Read the model definition and answer for the solid it produces. Units are mm, in the model's axes. A direction names the side the tool comes from. Coordinates: 2 decimals unless noted, no trailing zeros. Order: outer loops, then holes, each group sorted by start corner. A loop starts at its lowest first (then second) coordinate and runs counter-clockwise, first axis right, second up.
```python
from build123d import *

# Parameters (mm, degrees)
BOSS_EXTRUDE1_DEPTH    = 2
FILLET1_R              = 1
SKETCH2_R              = 1.65
BOSS_EXTRUDE2_DEPTH    = 2
CONVERT_SOLID1_START   = -25
CONVERT_SOLID1_DEPTH   = 25
CONVERT_SOLID1_2_DEPTH = 25


# Read off the part's stored shape, not the designer's step: Convert-Solid1
with BuildPart() as part:
    # Sketch1 → Boss-Extrude1 (new body)
    with BuildSketch(Plane(origin=(0, 0, 0), x_dir=(1, 0, 0), z_dir=(0, 1, 0))):
        with BuildLine():
            Line((51, 12.5), (47.9, 12.5))
            ThreePointArc((47.9, 12.5), (46.4, 11), (44.9, 12.5))
            Line((44.9, 12.5), (41.7, 12.5))
            ThreePointArc((41.7, 12.5), (40.2, 11), (38.7, 12.5))
            Line((38.7, 12.5), (35.5, 12.5))
            ThreePointArc((35.5, 12.5), (34, 11), (32.5, 12.5))
            Line((32.5, 12.5), (29.3, 12.5))
            ThreePointArc((29.3, 12.5), (27.8, 11), (26.3, 12.5))
            Line((26.3, 12.5), (23.1, 12.5))
            ThreePointArc((23.1, 12.5), (21.6, 11), (20.1, 12.5))
            Line((20.1, 12.5), (16.9, 12.5))
            ThreePointArc((16.9, 12.5), (15.4, 11), (13.9, 12.5))
            Line((13.9, 12.5), (10.7, 12.5))
            ThreePointArc((10.7, 12.5), (9.2, 11), (7.7, 12.5))
            Line((7.7, 12.5), (0, 12.5))
            Line((0, 12.5), (0, 0))
            Line((0, 0), (4.7, 0))
            Line((4.7, 0), (4.7, 1.5))
            ThreePointArc((4.7, 1.5), (6.2, 3), (7.7, 1.5))
            Line((7.7, 1.5), (7.7, 0))
            Line((7.7, 0), (10.9, 0))
            Line((10.9, 0), (10.9, 1.5))
            ThreePointArc((10.9, 1.5), (12.4, 3), (13.9, 1.5))
            Line((13.9, 1.5), (13.9, 0))
            Line((13.9, 0), (17.1, 0))
            Line((17.1, 0), (17.1, 1.5))
            ThreePointArc((17.1, 1.5), (18.6, 3), (20.1, 1.5))
            Line((20.1, 1.5), (20.1, 0))
            Line((20.1, 0), (23.3, 0))
            Line((23.3, 0), (23.3, 1.5))
            ThreePointArc((23.3, 1.5), (24.8, 3), (26.3, 1.5))
            Line((26.3, 1.5), (26.3, 0))
            Line((26.3, 0), (29.5, 0))
            Line((29.5, 0), (29.5, 1.5))
            ThreePointArc((29.5, 1.5), (31, 3), (32.5, 1.5))
            Line((32.5, 1.5), (32.5, 0))
            Line((32.5, 0), (35.7, 0))
            Line((35.7, 0), (35.7, 1.5))
            ThreePointArc((35.7, 1.5), (37.2, 3), (38.7, 1.5))
            Line((38.7, 1.5), (38.7, 0))
            Line((38.7, 0), (41.9, 0))
            Line((41.9, 0), (41.9, 1.5))
            ThreePointArc((41.9, 1.5), (43.4, 3), (44.9, 1.5))
            Line((44.9, 1.5), (44.9, 0))
            Line((44.9, 0), (46.5, 0))
            ThreePointArc((46.5, 0), (49.681980515, 1.318019485), (51, 4.5))
            Line((51, 4.5), (51, 12.5))
        make_face()
        with BuildLine():
            ThreePointArc((44.9, 12.5), (46.4, 14), (47.9, 12.5))
            Line((47.9, 12.5), (51, 12.5))
            Line((51, 12.5), (51, 20.5))
            ThreePointArc((51, 20.5), (49.681980515, 23.681980515), (46.5, 25))
            Line((46.5, 25), (44.9, 25))
            Line((44.9, 25), (44.9, 23.5))
            ThreePointArc((44.9, 23.5), (43.4, 22), (41.9, 23.5))
            Line((41.9, 23.5), (41.9, 25))
            Line((41.9, 25), (38.7, 25))
            Line((38.7, 25), (38.7, 23.5))
            ThreePointArc((38.7, 23.5), (37.2, 22), (35.7, 23.5))
            Line((35.7, 23.5), (35.7, 25))
            Line((35.7, 25), (32.5, 25))
            Line((32.5, 25), (32.5, 23.5))
            ThreePointArc((32.5, 23.5), (31, 22), (29.5, 23.5))
            Line((29.5, 23.5), (29.5, 25))
            Line((29.5, 25), (26.3, 25))
            Line((26.3, 25), (26.3, 23.5))
            ThreePointArc((26.3, 23.5), (24.8, 22), (23.3, 23.5))
            Line((23.3, 23.5), (23.3, 25))
            Line((23.3, 25), (20.1, 25))
            Line((20.1, 25), (20.1, 23.5))
            ThreePointArc((20.1, 23.5), (18.6, 22), (17.1, 23.5))
            Line((17.1, 23.5), (17.1, 25))
            Line((17.1, 25), (13.9, 25))
            Line((13.9, 25), (13.9, 23.5))
            ThreePointArc((13.9, 23.5), (12.4, 22), (10.9, 23.5))
            Line((10.9, 23.5), (10.9, 25))
            Line((10.9, 25), (7.7, 25))
            Line((7.7, 25), (7.7, 23.5))
            ThreePointArc((7.7, 23.5), (6.2, 22), (4.7, 23.5))
            Line((4.7, 23.5), (4.7, 25))
            Line((4.7, 25), (0, 25))
            Line((0, 25), (0, 12.5))
            Line((0, 12.5), (7.7, 12.5))
            ThreePointArc((7.7, 12.5), (9.2, 14), (10.7, 12.5))
            Line((10.7, 12.5), (13.9, 12.5))
            ThreePointArc((13.9, 12.5), (15.4, 14), (16.9, 12.5))
            Line((16.9, 12.5), (20.1, 12.5))
            ThreePointArc((20.1, 12.5), (21.6, 14), (23.1, 12.5))
            Line((23.1, 12.5), (26.3, 12.5))
            ThreePointArc((26.3, 12.5), (27.8, 14), (29.3, 12.5))
            Line((29.3, 12.5), (32.5, 12.5))
            ThreePointArc((32.5, 12.5), (34, 14), (35.5, 12.5))
            Line((35.5, 12.5), (38.7, 12.5))
            ThreePointArc((38.7, 12.5), (40.2, 14), (41.7, 12.5))
            Line((41.7, 12.5), (44.9, 12.5))
        make_face()
    extrude(amount=BOSS_EXTRUDE1_DEPTH)

    # Fillet1
    fillet1_edges = [part.edges().sort_by_distance(p)[0] for p in [
        (44.9, 1, 0),
        (41.9, 1, 0),
        (38.7, 1, 0),
        (35.7, 1, 0),
        (32.5, 1, 0),
        (29.5, 1, 0),
        (26.3, 1, 0),
        (23.3, 1, 0),
        (20.1, 1, 0),
        (17.1, 1, 0),
        (13.9, 1, 0),
        (10.9, 1, 0),
        (7.7, 1, 0),
        (4.7, 1, 0),
        (4.7, 1, -25),
        (7.7, 1, -25),
        (10.9, 1, -25),
        (13.9, 1, -25),
        (17.1, 1, -25),
        (20.1, 1, -25),
        (23.3, 1, -25),
        (26.3, 1, -25),
        (29.5, 1, -25),
        (32.5, 1, -25),
        (35.7, 1, -25),
        (38.7, 1, -25),
        (41.9, 1, -25),
        (44.9, 1, -25),
    ]]
    fillet(fillet1_edges, radius=FILLET1_R)

    # Sketch2 → Boss-Extrude2 (add)
    # profile 1 of 3: a face of its own
    with BuildSketch(Plane(origin=(0, 0, 0), x_dir=(0, 0, -1), z_dir=(1, 0, 0))):
        with BuildLine():
            Line((0, 0), (25, 0))
            Line((25, 0), (25, 14.5))
            ThreePointArc((25, 14.5), (12.5, 2), (0, 14.5))
            Line((0, 14.5), (0, 0))
        make_face()
    # profile 2 of 3: a face of its own
    with BuildSketch(Plane(origin=(0, 0, 0), x_dir=(0, 0, -1), z_dir=(1, 0, 0))):
        with BuildLine():
            ThreePointArc((0, 14.5), (12.5, 2), (25, 14.5))
            Line((25, 14.5), (22.65, 14.5))
            ThreePointArc((22.65, 14.5), (21, 12.85), (19.35, 14.5))
            Line((19.35, 14.5), (16.25, 14.5))
            ThreePointArc((16.25, 14.5), (12.5, 10.75), (8.75, 14.5))
            Line((8.75, 14.5), (5.65, 14.5))
            ThreePointArc((5.65, 14.5), (4, 12.85), (2.35, 14.5))
            Line((2.35, 14.5), (0, 14.5))
        make_face()
        with Locations((12.5, 6)):
            Circle(SKETCH2_R, mode=Mode.SUBTRACT)
    # profile 3 of 3: a face of its own
    with BuildSketch(Plane(origin=(0, 0, 0), x_dir=(0, 0, -1), z_dir=(1, 0, 0))):
        with BuildLine():
            Line((22.65, 14.5), (25, 14.5))
            ThreePointArc((25, 14.5), (12.5, 27), (0, 14.5))
            Line((0, 14.5), (2.35, 14.5))
            ThreePointArc((2.35, 14.5), (4, 16.15), (5.65, 14.5))
            Line((5.65, 14.5), (8.75, 14.5))
            ThreePointArc((8.75, 14.5), (12.5, 18.25), (16.25, 14.5))
            Line((16.25, 14.5), (19.35, 14.5))
            ThreePointArc((19.35, 14.5), (21, 16.15), (22.65, 14.5))
        make_face()
        with Locations((12.5, 23)):
            Circle(SKETCH2_R, mode=Mode.SUBTRACT)
    extrude(amount=BOSS_EXTRUDE2_DEPTH)

    # Convert-Solid1 outline → Convert-Solid1 (cut)
    with BuildSketch(Plane.XY.offset(CONVERT_SOLID1_START)):
        with BuildLine():
            ThreePointArc((3, 0), (0.878679656, 0.878679656), (0, 3))
            Line((0, 3), (0, 0))
            Line((0, 0), (3, 0))
        make_face()
    extrude(amount=CONVERT_SOLID1_DEPTH, mode=Mode.SUBTRACT)

    # Convert-Solid1 2 outline → Convert-Solid1 2 (add)
    with BuildSketch(Plane.XY.offset(CONVERT_SOLID1_START)):
        with BuildLine():
            ThreePointArc((3, 2), (2.292893219, 2.292893219), (2, 3))
            Line((2, 3), (2, 2))
            Line((2, 2), (3, 2))
        make_face()
    extrude(amount=CONVERT_SOLID1_2_DEPTH)


solid = part.part
```
1) A cutting plane is placed at B-B, the plane z = -9.75. Determine the outline of the cut face in (x, y).
A:
outline: (0, 3) arc R3 ccw to (3, 0) - (51, 0) - (51, 2) - (3, 2) arc R1 cw to (2, 3) - (2, 11.95) - (0, 11.95) - close; (0, 17.05) - (2, 17.05) - (2, 26.69) - (0, 26.69) - close
2) Flat-ended cylindrical pins translate along their axes: pin 1 Ø2 at (y, z) = (23, -12.5) entering from +X; pin 2 Ø1.5 at (x, z) = (38, -20) entering from +Y; pin 3 Ø10 at (y, z) = (9, -16.5) entering from -X; pin 4 Ø0.6 at (y, z) = (1, -1.5) entering from +X. Find the tip coordinate at first contact, or state that the pin passes through.
A:
pin 1: passes through
pin 2: stops at y = 2
pin 3: stops at x = 0
pin 4: stops at x = 50.1
3) Which of the six approach directions +Z, -Z, +X, -X, +Y, -Y give full straight-line access (tool end or side, diameter ignored) to faces 1 (the cylindrical face through (26.37, 0.99, -12.95)), 2 (the cylindrical face through (16.799, 1.014, -0.285)), 3 (the cylindrical face through (39.001, 1.014, -24.715))?
A:
face 1: +Y, -Y
face 2: +Z, +Y, -Y
face 3: -Z, +Y, -Y
4) A cutting plane is placed at D-D, the plane z = -12.5. State how many separate pieces and enclosed holes the cut face has, and give its area (3 significant figures).
A:
separate pieces: 11
enclosed holes: 0
area: 80.1 mm2
5) A cutting plane is placed at C-C, the plane x = 24.8. Determine the outline of the cut face in (y, z), and give its area (3 significant figures).
A:
outline: (0, -22) - (2, -22) - (2, -3) - (0, -3) - close
area: 38.0 mm2
6) A cutting plane is placed at A-A, the plane y = 6. Determine the outline of the cut face in (x, z), and give its area (3 significant figures).
A:
outline: (0, -25) - (2, -25) - (2, -14.15) - (0, -14.15) - close; (0, -10.85) - (2, -10.85) - (2, 0) - (0, 0) - close
area: 43.4 mm2
7) Determine the mould class of faces 4 (the cylindrical face through (0.986, 16.782, -9.524)), 5 (the cylindrical face through (0.9, 0.86, -12.68)), 6 (the cylindrical face through (24.8, 1, -22)) for opening direction X: pulls with the +X half, pulls with the -X half, needs draft (parallel to the pull), parting line crosses it, or undercut.
A:
face 4: needs draft
face 5: pulls with the -X half
face 6: undercut
8) Straight lines are drawn through the part: line 1 (Z direction, x = 1.25, y = 14.5); line 2 (Z direction, x = 15.4, y = 0.7); line 3 (Y direction, x = 0.4, z = -12.5). For each, find the intervals that lie inside material, in ascending order.
A:
line 1: z = -25 to -22.65, -19.35 to -16.25, -8.75 to -5.65, -2.35 to 0
line 2: z = -25 to -14, -11 to 0
line 3: y = 1.5 to 4.35, 7.65 to 10.75, 18.25 to 21.35, 24.65 to 27
